Can you work these out from the model? Positions are in its coordinate system, mm. Face numbers are marked on the shaded views. Round coordinates to 2 decimals unless told otherwise and drop trailing zeros. Write each loop counter-clockwise with the first axis right and the second up, starting at its lowest first coordinate (ties: lowest second). Pieces come first, ordered by that corner, then holes. Notation, with made-up numbers: M 77,19 L 126,19 A20 cw 126,24 Z; hole C -2.5,87.25 d10. An arc over 180 degrees is marked long. Answer in a Markdown table with one row per item. Add a question column.
(1) If I drill on probe 1 along Z at (x, y) = (4.5, 15.25); probe 2 along X at (y, z) = (9.25, 2.15); probe 3 along X at (y, z) = (11.5, 0.7), over which ranges is the centre line in solid material (lowest first)?
(2) I'm going to push a flat-ended pin straight in: pin 1 (1 mm diameter, centred on x = 4, y = 12, fed in from -Z). Where does the tip first touch, or does it pass through?
(3) If we mould it in two halves opening along X, with no side actions, what happens to the marked faces 1, 2, 3 and 4? For each: released by +X, released by -X, zero draft, split by the parting line, or undercut.
(4) Suppose I cut it at C-C, the plane z = 0.55. Write out the boundary of the cut face in (x, y).
(5) Suppose I cut it at B-B, the plane x = 1. Write out the boundary of the cut face in (y, z).
(6) Suppose I cut it at A-A, the plane y = 11. Write out the boundary of the cut face in (x, z).
(7) Suppose I cut it at D-D, the plane x = 3.5. Write out the boundary of the cut face in (y, z), then the cut area to 3 significant figures.
from build123d import *

# Parameters (mm, degrees)
F0_W      = 14
F0_H      = 9
F1_DEPTH  = 1
F2_R      = 2.75
F2_R_2    = 2.1
F3_DEPTH  = 2
F3_FACE_R = 2.1
F4_DEPTH  = 1.5
F5_R      = 2
F7_DEPTH  = 25


with BuildPart() as f1:
    # F0 (on Top) → F1 (new body)
    with BuildSketch(Plane.XY):
        with Locations((0.901556, 11.815395)):
            Rectangle(F0_W, F0_H)
    extrude(amount=F1_DEPTH)

    # F2 (on face) → F3 (join)
    with BuildSketch(Plane.XY.offset(1)):
        with Locations((0.901556, 10.815395)):
            Circle(F2_R)
        with Locations((0.901556, 10.815395)):
            Circle(F2_R_2, mode=Mode.SUBTRACT)
    extrude(amount=F3_DEPTH)

    # F3_face (on face) → F4 (cut)
    with BuildSketch(Plane(origin=(0.901556, 10.815395, 1), x_dir=(1, 0, 0), z_dir=(0, 0, 1))):
        Circle(F3_FACE_R)
    extrude(amount=-F4_DEPTH, mode=Mode.SUBTRACT)

    # F5
    f5_edges = [f1.edges().sort_by_distance(p)[0] for p in [
        (-6.098444, 7.315395, 0.5),
        (-6.098444, 16.315395, 0.5),
        (7.901556, 7.315395, 0.5),
        (7.901556, 16.315395, 0.5),
    ]]
    fillet(f5_edges, radius=F5_R)

    # F6 (on face) → F7 (cut)
    with BuildSketch(Plane.XZ.offset(-7.315395)):
        Polygon((0.521946, 3.445374), (-2.167966, 3.445374), (-2.167966, 1), align=None)
    extrude(amount=-F7_DEPTH, mode=Mode.SUBTRACT)


solid = f1.part
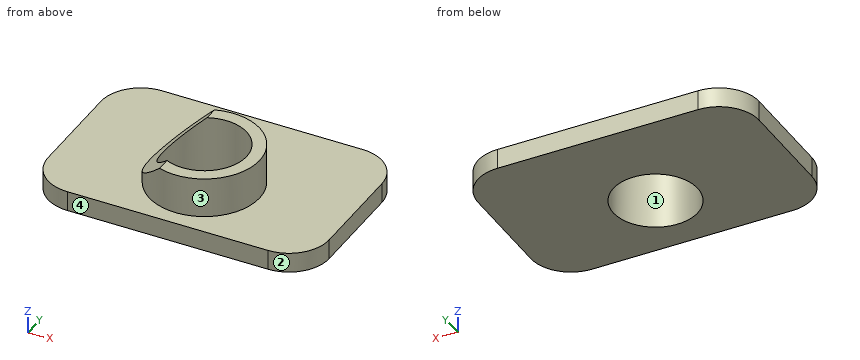
Calculated:
| question | item | result |
|---|---|---|
| 1 | probe 1 | 0 to 1 |
| 1 | probe 2 | -0.9 to -0.5, 2.3 to 3.16 |
| 1 | probe 3 | -6.1 to -1.08, 2.89 to 7.9 |
| 2 | pin 1 | z = 0 |
| 3 | face 1 | undercut |
| 3 | face 2 | released by +X |
| 3 | face 3 | split by the parting line |
| 3 | face 4 | zero draft |
| 4 | outline | M -6.1,9.32 A2 ccw -4.1,7.32 L 5.9,7.32 A2 ccw 7.9,9.32 L 7.9,14.32 A2 ccw 5.9,16.32 L -4.1,16.32 A2 ccw -6.1,14.32 Z; hole C 0.9,10.82 d4.2 |
| 5 | outline | M 7.32,0 L 8.72,0 L 8.72,3 L 8.07,3 L 8.07,1 L 7.32,1 Z; M 12.91,0 L 16.32,0 L 16.32,1 L 13.56,1 L 13.56,3 L 12.91,3 Z |
| 6 | outline | M -6.1,0 L -1.19,0 L -1.19,1.89 L -1.84,1.3 L -1.84,1 L -6.1,1 Z; M 2.99,0 L 7.9,0 L 7.9,1 L 3.65,1 L 3.65,3 L 2.99,3 Z |
| 7 | outline | M 7.32,0 L 16.32,0 L 16.32,1 L 11.72,1 L 11.72,3 L 9.92,3 L 9.92,1 L 7.32,1 Z |
| 7 | area | 12.6 mm² |
